Source: three-view drawing plus pictorial views. Frame: mm from the lowest corner of the part. A direction names the side the tool comes from. Give positions to 0.01 mm unless a question says otherwise; leave off trailing zeros. Loops run counter-clockwise (first coordinate to the right, second up) from the corner with the lowest first, then second, coordinate; pieces in that order, holes last.
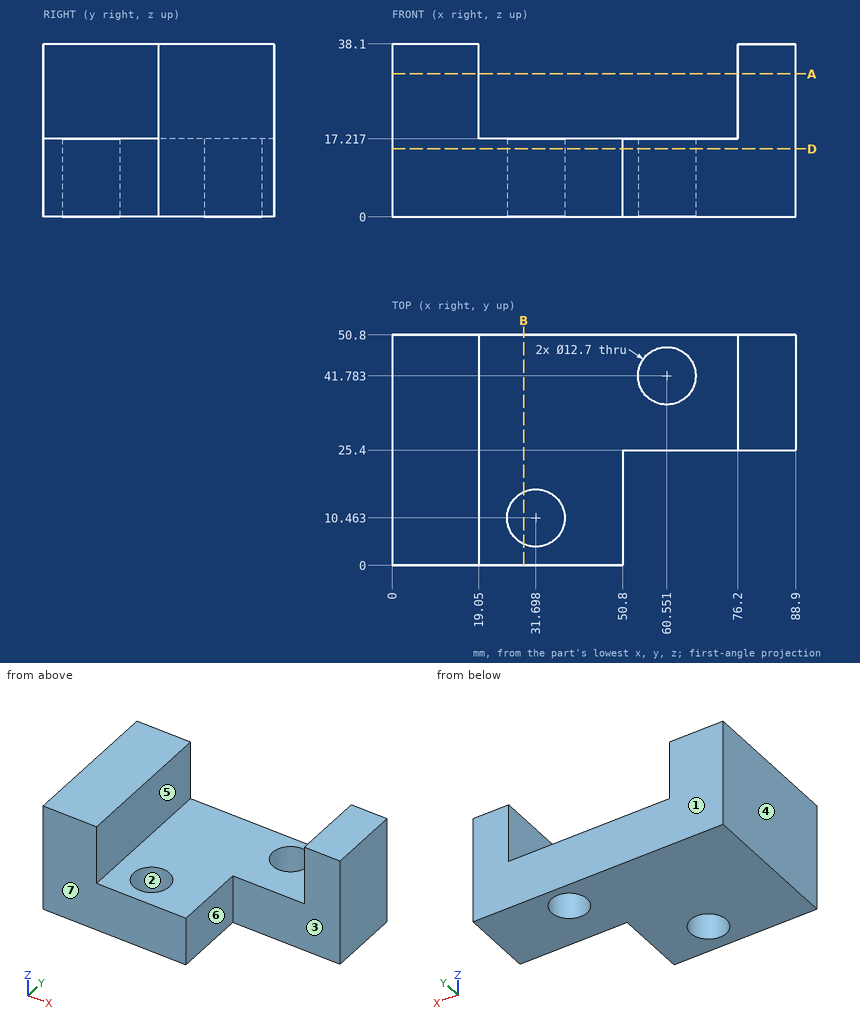
Q1. Section query D-D, the plane z = 15. Return loops of the section in (x, y).
Q2. Material intervals for probe 1 along X at (y, z) = (27.5, 32); probe 2 along Z at (x, y) = (25, 18); probe 3 along Y at (x, z) = (32.5, 9), sorted ascending.
Q3. Section query B-B, the plane x = 29. Return loops of the section in (y, z) (1 decimal).
Q4. Pin query (flat end, axial travel): pin 1 Ø19 at (y, z) = (11.5, 11.5) entering from +X; pin 2 Ø5 at (x, y) = (28, 34) entering from +Z; pin 3 Ø5 at (x, z) = (68, 22) entering from +Y; pin 4 Ø4 at (y, z) = (18.5, 23.5) entering from +X. Return the tip coordinate at first contact, or that it passes through.
Q5. Mould query, pull axis Y, two halves, no side actions, for the marked faces 1, 2, 3 and 4. Classes: +Y half, -Y half, draft (parallel to the pull), parting line (faces both ways), or undercut.
Q6. Section query A-A, the plane z = 31.5. Return loops of the section in (x, y).
Q7. Reachability of the marked faces 5, 6 and 7 from +Z, -Z, +X, -X, +Y, -Y: full face, straight path, thin tool, end or side. Return the list, or none.
Resolved:
1. outline: (0, 0) - (50.8, 0) - (50.8, 25.4) - (88.9, 25.4) - (88.9, 50.8) - (0, 50.8) - close; hole circle Ø12.7 at (31.7, 10.46); hole circle Ø12.7 at (60.55, 41.78)
2. probe 1: x = 0 to 19.05, 76.2 to 88.9
2. probe 2: z = 0 to 17.22
2. probe 3: y = 0 to 4.16, 16.76 to 50.8
3. outline: (0, 0) - (4.7, 0) - (4.7, 17.2) - (0, 17.2) - close; (16.2, 0) - (50.8, 0) - (50.8, 17.2) - (16.2, 17.2) - close
4. pin 1: stops at x = 50.8
4. pin 2: stops at z = 17.22
4. pin 3: passes through
4. pin 4: stops at x = 19.05
5. face 1: +Y half
5. face 2: undercut
5. face 3: -Y half
5. face 4: draft
6. outline: (0, 0) - (19.05, 0) - (19.05, 50.8) - (0, 50.8) - close; (76.2, 25.4) - (88.9, 25.4) - (88.9, 50.8) - (76.2, 50.8) - close
7. face 5: +Z, +Y, -Y
7. face 6: +Z, -Z, +X, -Y
7. face 7: +Z, -Z, +X, -X, -Y
